```python
from build123d import *

# Parameters (mm, degrees)
F0_W      = 40
F0_H      = 25
F1_DEPTH  = 3
F2_R      = 5
F3_W      = 52
F3_H      = 25
F4_DEPTH  = 2
F5_R      = 3
F6_R      = 1.5
F7_DEPTH  = 25
F8_R      = 1.5
F9_DEPTH  = 4
F10_W     = 24
F10_H     = 25
F11_DEPTH = 3
F12_W     = 4
F12_H     = 16
F12_R     = 4
F13_DEPTH = 25
F14_R     = 1.99999


# Not quite as in the source:
# - a fillet or chamfer is up to 0.001 mm smaller than in the source, because OpenCascade refuses the exact size


with BuildPart() as f1:
    # F0 (on Top) → F1 (new body)
    with BuildSketch(Plane.XY):
        Rectangle(F0_W, F0_H)
    extrude(amount=F1_DEPTH)

    # F2
    f2_edges = [f1.edges().sort_by_distance(p)[0] for p in [
        (-20, -12.5, 1.5),
        (-20, 12.5, 1.5),
        (20, -12.5, 1.5),
        (20, 12.5, 1.5),
    ]]
    fillet(f2_edges, radius=F2_R)

    # F3 (on face) → F4 (join)
    with BuildSketch(Plane.XY.offset(3)):
        Rectangle(F3_W, F3_H)
    extrude(amount=F4_DEPTH)

    # F5
    f5_edges = [f1.edges().sort_by_distance(p)[0] for p in [
        (26, 12.5, 4),
        (26, -12.5, 4),
        (-26, -12.5, 4),
        (-26, 12.5, 4),
    ]]
    fillet(f5_edges, radius=F5_R)

    # F6 (on Top) → F7 (cut)
    with BuildSketch(Plane.XY):
        with Locations((23, 9)):
            Circle(F6_R)
        with Locations((23, -9)):
            Circle(F6_R)
        with Locations((-23, -9)):
            Circle(F6_R)
        with Locations((-23, 9)):
            Circle(F6_R)
    extrude(amount=F7_DEPTH, mode=Mode.SUBTRACT)

    # F8 (on face) → F9 (cut)
    with BuildSketch(Plane.XY.offset(5)):
        with Locations((16, -9)):
            Circle(F8_R)
        with Locations((-16, -9)):
            Circle(F8_R)
        with Locations((-16, 9)):
            Circle(F8_R)
        with Locations((16, 9)):
            Circle(F8_R)
    extrude(amount=-F9_DEPTH, mode=Mode.SUBTRACT)

    # F10 (on face) → F11 (cut)
    with BuildSketch(Plane.XY.offset(5)):
        Rectangle(F10_W, F10_H)
    extrude(amount=-F11_DEPTH, mode=Mode.SUBTRACT)

    # F12 (on face) → F13 (cut)
    with BuildSketch(Plane(origin=(0, 0, 0), x_dir=(1, 0, 0), z_dir=(0, 0, -1))):
        with Locations((7, 0)):
            Rectangle(F12_W, F12_H)
        with Locations((-6, -6)):
            Circle(F12_R)
        with Locations((-6, 6)):
            Circle(F12_R)
    extrude(amount=-F13_DEPTH, mode=Mode.SUBTRACT)

    # F14 (radius 2 in the source; OpenCascade refuses exactly that, so slightly less here)
    f14_edges = [f1.edges().sort_by_distance(p)[0] for p in [
        (9, 8, 1),
        (5, 8, 1),
        (9, -8, 1),
        (5, -8, 1),
    ]]
    fillet(f14_edges, radius=F14_R)


solid = f1.part
```
Geometry check sheet. Reference: the model listing, model coordinates, mm. A direction names the side the tool comes from. Give positions to 0.01 mm unless a question says otherwise; leave off trailing zeros. Order: outer loops, then holes, each group sorted by start corner. A loop starts at its lowest first (then second) coordinate and runs counter-clockwise, first axis right, second up.
1. Thickness scan on L1, parallel to X at y = -6, z = 0.4; L2, parallel to Y at x = -23, z = 3.65; L3, parallel to Y at x = -6, z = 1.15. Record the ranges inside material, lowest first.
2. Access from +Z, -Z, +X, -X, +Y, -Y to the whole of each face (thin tool, end or side, straight path). Record for faces 1 (the face through (14.8, -9.9, 3)), 2 (the face through (19, 0, 5)), 3 (the face through (5.57, 7.4, 1.01)).
3. Section check A-A, the plane x = -6. Enter the section's corners in (y, z), and give its area (3 significant figures).
4. Section check C-C, the plane y = -3.25. Enter the section's corners in (x, z), and give its area (3 significant figures).
5. Section check B-B, the plane z = 3.9. Give the number of separate pieces and of enclosed holes in the cut face, and give its area (3 significant figures).
6. Gauge pin test, flat ends, axial feed: pin 1 Ø0.9 at (x, y) = (-15.5, -9) entering from +Z; pin 2 Ø4 at (x, y) = (-5, -0.5) entering from +Z; pin 3 Ø4 at (x, y) = (-23, -9) entering from -Z. Record the tip position at first contact, or that the pin passes through.
7. Section check D-D, the plane x = 19. Enter the section's corners in (y, z).
8. Release check for a two-part mould opening along Y. For faces 4 (the face through (18.5, -11.07, 1.52)), 5 (the face through (23, 0, 3)), 6 (the face through (14.8, 8.1, 3)) record: pulls with the +Y half, pulls with the -Y half, needs draft (parallel to the pull), parting line crosses it, or undercut.
Values follow:
1. L1: x = -20 to -10, -2 to 5, 9 to 20
1. L2: y = -12.5 to -10.5, -7.5 to 7.5, 10.5 to 12.5
1. L3: y = -12.5 to -10, -2 to 2, 10 to 12.5
2. face 1: +Z
2. face 2: +Z, +X, -X, +Y, -Y
2. face 3: +Z, -Z
3. outline: (-12.5, 0) - (-10, 0) - (-10, 2) - (-12.5, 2) - close; (-2, 0) - (2, 0) - (2, 2) - (-2, 2) - close; (10, 0) - (12.5, 0) - (12.5, 2) - (10, 2) - close
3. area: 18.0 mm2
4. outline: (-26, 3) - (-20, 3) - (-20, 0) - (-8.9, 0) - (-8.9, 2) - (-12, 2) - (-12, 5) - (-26, 5) - close; (-3.1, 0) - (5, 0) - (5, 2) - (-3.1, 2) - close; (9, 0) - (20, 0) - (20, 3) - (26, 3) - (26, 5) - (12, 5) - (12, 2) - (9, 2) - close
4. area: 132 mm2
5. separate pieces: 2
5. enclosed holes: 8
5. area: 636 mm2
6. pin 1: stops at z = 1
6. pin 2: stops at z = 2
6. pin 3: stops at z = 3
7. outline: (-12.5, 3) - (-10.5, 3) - (-10.5, 0) - (10.5, 0) - (10.5, 3) - (12.5, 3) - (12.5, 5) - (-12.5, 5) - close
8. face 4: pulls with the -Y half
8. face 5: needs draft
8. face 6: undercut
